Check sheet for the drawn part. Datum: minimum x, y, z corner. Units: mm. A direction names the side the tool comes from. Coordinates: 2 decimals unless noted, no trailing zeros. Loops run counter-clockwise (first coordinate to the right, second up) from the corner with the lowest first, then second, coordinate; pieces in that order, holes last. Notation, with made-up numbers: (16.5, 79.5) -> (73.5, 79.5) arc R31 ccw to (73.5, 111.5) -> close; hole circle Ø5 at (42.25, 14). An arc over 180 degrees is marked (long way). Use CSV: the item, a comma, the result in double quotes. Start each with the question number.
1. Sectioned sample at B-B, the plane z = 25.4. Record the cut outline in (x, y).
2. Gauge pin test, flat ends, axial feed: pin 1 (3 mm diameter, centred on y = 3, z = 38, fed in from +X) (1 decimal); pin 2 (3 mm diameter, centred on x = 37.5, y = 5.5, fed in from +Z); pin 3 (3 mm diameter, centred on x = 16, y = 3.5, fed in from +Z). Record the tip position at first contact, or that the pin passes through.
3. Sectioned sample at C-C, the plane y = 7.25. Count the separate pieces of the cut face and the enclosed holes in it, and give its area (4 significant figures).
4. Set-up check for the marked faces 1 and 2: record each of +Z, -Z, +X, -X, +Y, -Y from which the full face is reachable in a straight line by a thin tool's end or side.
5. Thickness scan on L1, parallel to Z at x = 25.4, y = 6.5; L2, parallel to X at y = 6.5, z = 19 (1 decimal); L3, parallel to X at y = 3.5, z = 27.5 (1 decimal). Record the ranges inside material, lowest first.
6. Sectioned sample at A-A, the plane x = 25.4. Record the cut outline in (y, z).
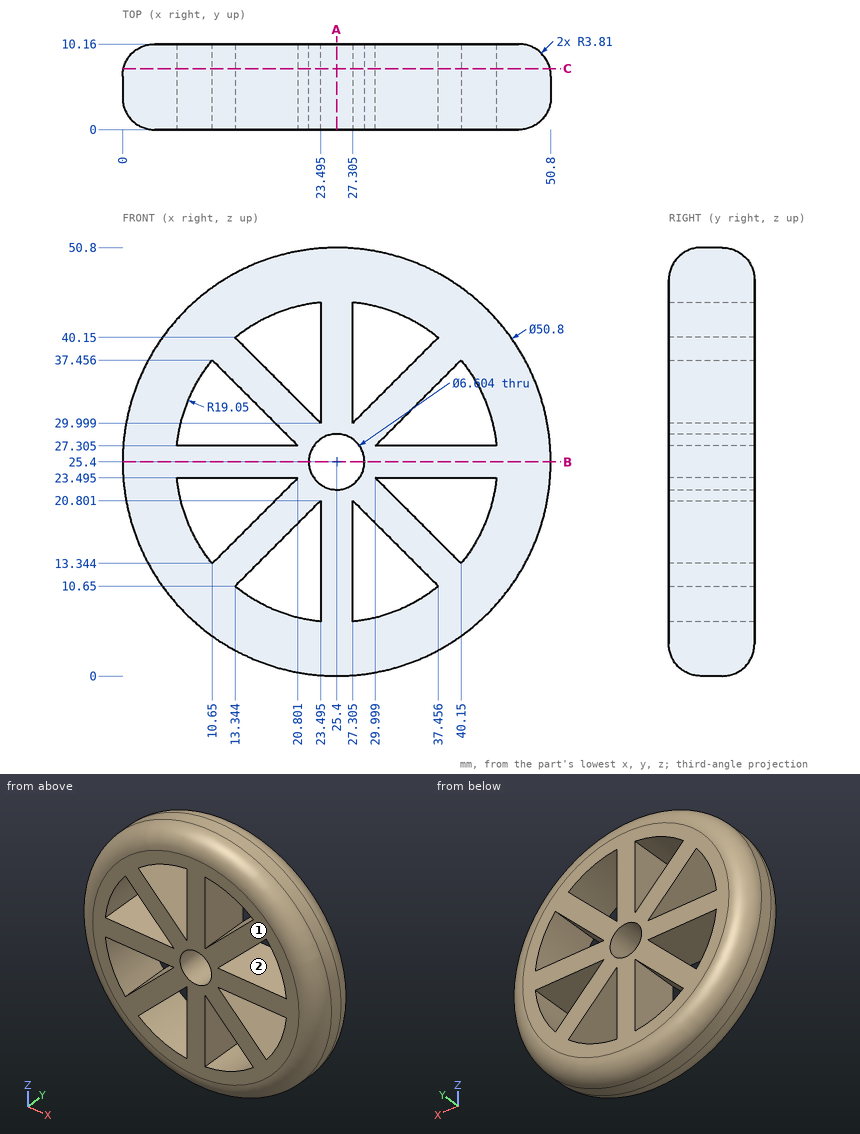
Completed:
1,outline,"(0, 3.81) arc R3.81 ccw to (3.81, 0) -> (22.1, 0) -> (22.1, 10.16) -> (3.81, 10.16) arc R3.81 ccw to (0, 6.35) -> close; (28.7, 0) -> (46.99, 0) arc R3.81 ccw to (50.8, 3.81) -> (50.8, 6.35) arc R3.81 ccw to (46.99, 10.16) -> (28.7, 10.16) -> close"
2,pin 1,"x = 48.2"
2,pin 2,"z = 48.48"
2,pin 3,"z = 49.53"
3,separate pieces,"1"
3,enclosed holes,"9"
3,area,"1,345 mm²"
4,face 1,"+Z, -Z, +X, -X, -Y"
4,face 2,"+Y, -Y"
5,L1,"0 to 22.1, 28.7 to 50.8"
5,L2,"0.8 to 7.5, 16.3 to 21.7, 23.5 to 27.3, 29.1 to 34.5, 43.3 to 50"
5,L3,"0.1 to 6.5, 20.6 to 22.9, 27.9 to 30.2, 44.3 to 50.7"
6,outline,"(0, 3.81) arc R3.81 ccw to (3.81, 0) -> (6.35, 0) arc R3.81 ccw to (10.16, 3.81) -> (10.16, 22.1) -> (0, 22.1) -> close; (0, 28.7) -> (10.16, 28.7) -> (10.16, 46.99) arc R3.81 ccw to (6.35, 50.8) -> (3.81, 50.8) arc R3.81 ccw to (0, 46.99) -> close"
